Autodesk Inventor part; units mm, degrees
ref_plane "YZ Plane" through (0, 0, 0) normal (1, 0, 0) x (0, 1, 0)
ref_plane "XZ Plane" through (0, 0, 0) normal (0, 1, 0) x (-1, 0, 0)
ref_plane "XY Plane" through (0, 0, 0) normal (0, 0, 1) x (1, 0, 0)
sketch "Sketch1" plane through (0, 0, 0) normal (0, 0, 1) x (1, 0, 0)
  line L0 (-9.398, 50.8) -> (9.398, 50.8)
  line L1 (9.398, 50.8) -> (9.398, -50.8)
  line L2 (9.398, -50.8) -> (-9.398, -50.8)
  line L3 (-9.398, -50.8) -> (-9.398, 50.8)
  line L4 (-9.398, 50.8) -> (9.398, -50.8) construction
  line L5 (9.398, 50.8) -> (-9.398, -50.8) construction
  point P0 (0, 0)
  dimension "d0" = 18.796
  dimension "d1" = 101.6
extrude "Extrusion1" add sketch "Sketch1" along normal mid plane 18.796
sketch "Sketch2" plane through (0, 0, 9.398) normal (0, 0, 1) x (1, 0, 0)
  line L0 (9.398, -50.8) -> (9.398, 50.8)
  line L1 (-9.398, -34.925) -> (9.398, -34.925)
  line L2 (9.398, -34.925) -> (9.398, -3.175)
  line L3 (9.398, -3.175) -> (-9.398, -3.175)
  line L4 (-9.398, -3.175) -> (-9.398, -34.925)
  line L5 (-9.398, -34.925) -> (9.398, -3.175) construction
  line L6 (9.398, -34.925) -> (-9.398, -3.175) construction
  line L7 (-9.398, -50.8) -> (9.398, -50.8)
  point P0 (0, 0)
  point P1 (0, -19.05)
  dimension "d4" = 31.75
  dimension "d5" = 15.875
  dimension "d6" = 18.796
extrude "Extrusion3" cut sketch "Sketch2" against normal blind 4.7498
sketch "Sketch3" plane through (0, 0, 4.6482) normal (0, 0, 1) x (1, 0, 0)
  circle A0 centre (0, -19.05) radius 3.9624
  line L0 (9.398, -34.925) -> (-9.398, -34.925)
  line L1 (9.398, -3.175) -> (9.398, -34.925)
  point P0 (0, 0)
  dimension "d11" = 7.9248
  dimension "d12" = 15.875
  dimension "d13" = 9.398
extrude "Extrusion4" cut sketch "Sketch3" against normal blind 15.24
sketch "Sketch4" plane through (0, 0, 9.398) normal (0, 0, 1) x (1, 0, 0)
  circle A0 centre (0, 41.275) radius 3.175
  line L0 (9.398, 50.8) -> (-9.398, 50.8)
  line L1 (9.398, -3.175) -> (9.398, 50.8)
  point P0 (0, 0)
  dimension "d16" = 6.35
  dimension "d17" = 9.525
  dimension "d18" = 9.398
extrude "Extrusion5" cut sketch "Sketch4" against normal blind 20.32
sketch "Sketch5" plane through (0, 0, 9.398) normal (0, 0, 1) x (1, 0, 0)
  circle A0 centre (-3.359, 22.225) radius 1.5875
  circle A1 centre (3.359, 22.225) radius 1.5875
  line L0 (9.398, 50.8) -> (-9.398, 50.8)
  line L1 (-9.398, 50.8) -> (9.398, 50.8)
  line L2 (0, 50.8) -> (0, -50.8) construction
  line L3 (9.398, -50.8) -> (-9.398, -50.8)
  circle A2 centre (0, 41.275) radius 3.175
  line L4 (0, 41.275) -> (3.359, 22.225) construction
  line L5 (0, 41.275) -> (-3.359, 22.225) construction
  point P0 (0, 0)
  dimension "d21" = 3.175
  dimension "d22" = 3.175
  dimension "d23" = 28.575
  dimension "d24" = 28.575
  dimension "d25" = 10
  dimension "d26" = 10
extrude "Extrusion6" cut sketch "Sketch5" against normal blind 20.32 contours A0
sketch "Sketch6" plane through (0, 0, 9.398) normal (0, 0, 1) x (1, 0, 0)
  circle A0 centre (-3.359, 22.225) radius 1.5875
  circle A1 centre (0, 41.275) radius 3.175
  circle A2 centre (3.359, 22.225) radius 1.5875
  line L0 (0, 41.275) -> (3.359, 22.225) construction
  line L1 (0, 41.275) -> (0, 8.045) construction
  line L2 (9.398, 50.8) -> (-9.398, 50.8)
  point P0 (0, 0)
  dimension "d29" = 3.175
  dimension "d31" = 10
  dimension "d32" = 28.575
extrude "Extrusion7" cut sketch "Sketch6" against normal blind 11.0998 contours A2
sketch "Sketch7" plane through (9.398, -50.8, -9.398) normal (1, 0, 0) x (0, 0, -1)
  line L0 (-18.796, 71.4375) -> (-18.796, 74.6125)
  circle A0 centre (-9.271, 73.025) radius 1.5875
  line L1 (0, 101.6) -> (0, 0)
  line L2 (-18.796, 101.6) -> (0, 101.6)
  point P0 (-9.398, 50.8)
  dimension "d35" = 3.175
  dimension "d36" = 9.271
  dimension "d37" = 28.575
extrude "Extrusion8" cut sketch "Sketch7" against normal blind 7.62
sketch "Sketch9" plane through (-9.398, -50.8, 9.398) normal (0, -1, 0) x (1, 0, 0)
  point P0 (9.398, -9.398)
  point P1 (9.398, -9.398)
hole "Hole1" at (0, -50.8, 0) direction (0, 1, 0) diameter 6.35 depth 19.05 tip angle 118
thread "Thread1"
equation "\"d24\" = d23"
equation "\"d26\" = d25"
properties part number "Standard"
Source: CAD feature listing. Evaluate the final solid. Frame: model axes, mm. A direction names the side the tool comes from. Coordinates: 2 decimals unless noted, no trailing zeros. Order: outer loops, then holes, each group sorted by start corner. A loop starts at its lowest first (then second) coordinate and runs counter-clockwise, first axis right, second up. Notation, with made-up numbers: M 50,-21.5 L 57,-21.5 A14 cw 57,-8.5 Z; hole C 13,-13.75 d4. An arc over 180 degrees is marked long. Write each question's results on one line, items separated by ' | '. Start each with the question number.
Item 1: Draft query along Y for faces 1 (the face through (0, -34.925, 7)), 2 (the face through (9.398, 1, 0)), 3 (the face through (-4, -50.8, 0)), 4 (the face through (0, 50.8, 0)). Return one class per face: pulls with the +Y half, pulls with the -Y half, needs draft (parallel to the pull), parting line crosses it, or undercut.
Item 2: Cut plane A-A (z = 6). Count the separate pieces of the cut face and the enclosed holes in it, and give its area (3 significant figures).
Item 3: Cut plane C-C (x = -7.5). Return loops of the section in (y, z) (3 decimals).
Item 4: Line query: probe 1 along Y at (x, z) = (0, 5.75) (3 decimals); probe 2 along Y at (x, z) = (2.25, 6) (3 decimals); probe 3 along Y at (x, z) = (0, -1.25). Output: solid intervals per line, ascending.
Item 5: First-contact query: pin 1 Ø7 at (x, y) = (0, -19.05) entering from -Z; pin 2 Ø1.1 at (x, y) = (3.5, 23) entering from +Z; pin 3 Ø10 at (x, y) = (-3.5, -28) entering from +Z; pin 4 Ø5 at (x, y) = (-3.359, 22.225) entering from -Z. Flat tips, straight axial feed; report the tip coordinate or a pass-through.
Item 6: Cut plane B-B (y = -40.5). Return loops of the section in (x, z) (3 decimals), and give its area (3 significant figures).
Item 7: Cut plane D-D (y = -19.05). Return loops of the section in (x, z), and give its area (3 significant figures).
Item 8: Set-up query: faces 5 (the face through (1.778, 21.9, -0.1)), 6 (the face through (0, -3.175, 7)), 7 (the face through (-0.52, -15.12, -2.28)), 8 (the face through (1.773, 22.295, 5.159)), 9 (the face through (3.1, -41.14, 0.69)). Return all of +Z, -Z, +X, -X, +Y, -Y with unobstructed straight access to the full face (end or side cutting, diameter ignored); none if empty.
Checked values:
1) face 1: undercut | face 2: needs draft | face 3: pulls with the -Y half | face 4: pulls with the +Y half
2) separate pieces: 2 | enclosed holes: 3 | area: 1,270 mm2
3) outline: M -50.8,-9.398 L 50.8,-9.398 L 50.8,9.398 L -3.175,9.398 L -3.175,4.648 L -34.925,4.648 L -34.925,9.398 L -50.8,9.398 Z
4) probe 1: y = -50.8 to -34.925, -3.175 to 38.1, 44.45 to 50.8 | probe 2: y = -50.8 to -34.925, -3.175 to 21.089, 23.361 to 39.035, 43.515 to 50.8 | probe 3: y = -30.59 to -23.01, -15.09 to 38.1, 44.45 to 50.8
5) pin 1: passes through | pin 2: stops at z = -1.7 | pin 3: stops at z = 4.65 | pin 4: stops at z = -9.4
6) outline: M -9.398,-9.398 L 9.398,-9.398 L 9.398,9.398 L -9.398,9.398 Z; hole C 0,0 d6.35 | area: 322 mm2
7) outline: M -9.4,-9.4 L -3.96,-9.4 L -3.96,4.65 L -9.4,4.65 Z; M 3.96,-9.4 L 9.4,-9.4 L 9.4,4.65 L 3.96,4.65 Z | area: 153 mm2
8) face 5: +X | face 6: +Z, +X, -X | face 7: +Z, -Z | face 8: +Z | face 9: -Y
